Geometry check sheet. Reference: drawing and pictorial views, mm from the part's lowest x, y, z. A direction names the side the tool comes from. Coordinates: 2 decimals unless noted, no trailing zeros. Write each loop counter-clockwise with the first axis right and the second up, starting at its lowest first coordinate (ties: lowest second). Pieces come first, ordered by that corner, then holes. Notation, with made-up numbers: (37, 69) -> (87, 69) arc R14 ccw to (87, 76) -> close; hole circle Ø8 at (81.5, -37). An arc over 180 degrees is marked (long way). Use a Markdown table: item, result.
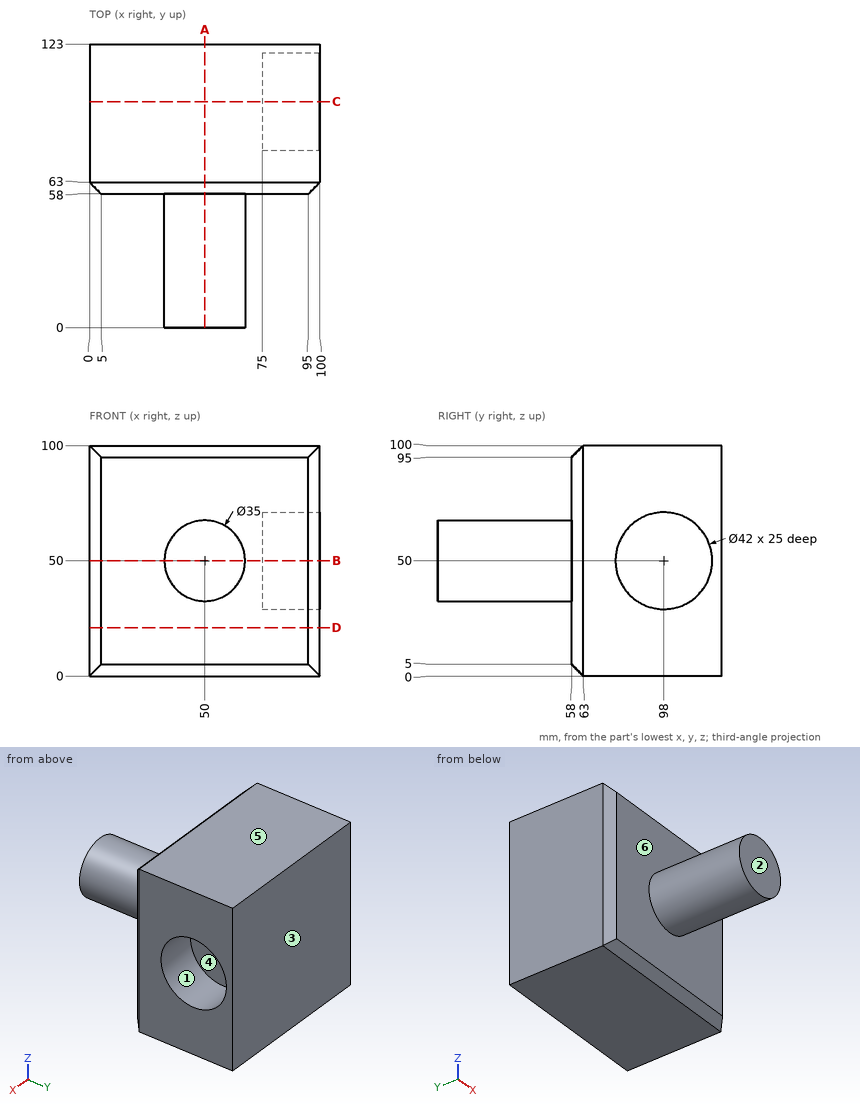
Item 1: Section check A-A on x = 50. Record the boundary of the cut face in (y, z), then the cut area to 4 significant figures.
Answer block:
| item | result |
|---|---|
| outline | (0, 32.5) -> (58, 32.5) -> (58, 5) -> (63, 0) -> (123, 0) -> (123, 100) -> (63, 100) -> (58, 95) -> (58, 67.5) -> (0, 67.5) -> close |
| area | 8,505 mm^2 |
Item 2: Section check B-B on z = 50. Record the boundary of the cut face in (x, y).
Answer block:
| item | result |
|---|---|
| outline | (0, 63) -> (5, 58) -> (32.5, 58) -> (32.5, 0) -> (67.5, 0) -> (67.5, 58) -> (95, 58) -> (100, 63) -> (100, 77) -> (75, 77) -> (75, 119) -> (100, 119) -> (100, 123) -> (0, 123) -> close |
Item 3: Section check C-C on y = 98. Record the boundary of the cut face in (x, z).
Answer block:
| item | result |
|---|---|
| outline | (0, 0) -> (100, 0) -> (100, 29) -> (75, 29) -> (75, 71) -> (100, 71) -> (100, 100) -> (0, 100) -> close |
Item 4: Thickness scan on L1, parallel to Z at x = 81, y = 98; L2, parallel to Y at x = 28.5, z = 67; L3, parallel to X at y = 99.5, z = 55. Record the ranges inside material, lowest first. Write a range as [from, to].
Answer block:
| item | result |
|---|---|
| L1 | z = [0, 29], [71, 100] |
| L2 | y = [58, 123] |
| L3 | x = [0, 75] |
Item 5: Tool access check on the marked faces 5 and 6. Record the directions out of +Z, -Z, +X, -X, +Y, -Y that give a thin tool (end or side, any length) a straight path to the whole face; none if there is none.
Answer block:
| item | result |
|---|---|
| face 5 | +Z, +X, -X, +Y, -Y |
| face 6 | -Y |
Item 6: Section check D-D on z = 21. Record the boundary of the cut face in (x, y), then the cut area to 4 significant figures.
Answer block:
| item | result |
|---|---|
| outline | (0, 63) -> (5, 58) -> (95, 58) -> (100, 63) -> (100, 123) -> (0, 123) -> close |
| area | 6,475 mm^2 |
Item 7: Depth check by flat-ended pin: P1, Ø1.5, axis at y = 14, z = 37, coming from the +X side; P2, Ø1.5, axis at y = 35.5, z = 38, coming from the +X side. Enter the tip coordinate at first touch or a pass-through.
Answer block:
| item | result |
|---|---|
| P1 | stops at x = 62.5 |
| P2 | stops at x = 63.4 |
Item 8: Mould release check, pull along Y, two halves, no side actions. Record for the marked faces 1, 2, 3 and 4: +Y half, -Y half, draft (parallel to the pull), parting line (faces both ways), or undercut.
Answer block:
| item | result |
|---|---|
| face 1 | undercut |
| face 2 | -Y half |
| face 3 | +Y half |
| face 4 | undercut |
